Autodesk Inventor part; units mm, degrees
ref_plane "Work Plane1" through (0, -14.5, 0) normal (0, 1, 0) x (-1, 0, 0)
ref_plane "Work Plane2" through (0, 14.5, 0) normal (0, 1, 0) x (-1, 0, 0)
ref_plane "YZ Plane" through (0, 0, 0) normal (1, 0, 0) x (0, 1, 0)
sketch "Sketch2" plane through (0, 0, 0) normal (0, 1, 0) x (-1, 0, 0)
  circle A0 centre (-25, -83.5) radius 36 construction
  line L0 (-25, -83.5) -> (-61, -83.5) construction
  line L1 (-25, -83.5) -> (4.6941, -63.1466) construction
  circle A1 centre (-25, -83.5) radius 41.5
  circle A2 centre (-25, -83.5) radius 28
  arc A3 (-8.1325, -61.1508) -> (0, -50.3752) centre (-4.0663, -55.763) ccw
  arc A4 (-50, -50.3752) -> (-39.3017, -57.0193) centre (-45.9337, -55.763) ccw
  line L2 (-25, -83.5) -> (-4.0663, -55.763) construction
  circle A5 centre (-25, -83.5) radius 31.5
  line L3 (0, -50.3752) -> (0, 0)
  line L4 (-50, -50.3752) -> (-50, 0)
  line L5 (0, 0) -> (-50, 0)
  line L6 (-25, 0) -> (-25, -83.5) construction
  point P0 (15.9829, -76.969)
  point P1 (13.8342, -68.866)
  point P2 (-39.2078, -55.1936)
  point P3 (-41.8675, -61.1508)
  point P4 (-8.1325, -61.1508)
  dimension "d1" = 72
  dimension "d5" = 83
  dimension "d6" = 56
  dimension "d7" = 63
  dimension "d11" = 50
  dimension "d31" = 83.5
ref_plane "Work Plane1" through (0, -14.5, 0) normal (0, 1, 0) x (-1, 0, 0)
ref_plane "Work Plane2" through (0, 14.5, 0) normal (0, 1, 0) x (-1, 0, 0)
extrude "Extrusion1" add sketch "Sketch2" along normal blind 12 from surface at 14.5 contours A1 A4 A5 A3 | A3 A5 A4 A1
extrude "Extrusion2" add sketch "Sketch2" against normal blind 12 from surface at -14.5 contours A3 A5 A4 A1 | A3 A2 A4 A5 picked at (-44.9519, -51.1635) picked at (-38.3765, -56.444)
extrude "Extrusion3" add sketch "Sketch2" along normal mid plane 53 contours A1 L4 L5 L3
sketch "Sketch3" plane through (0, 0, 0) normal (1, 0, 0) x (0, 1, 0)
  line L0 (26.5, 0) -> (-26.5, 0)
  circle A0 centre (0, 0) radius 26.5
extrude "Extrusion4" add sketch "Sketch3" along normal up to surface (50 mm away)
properties part number "left_thigh"
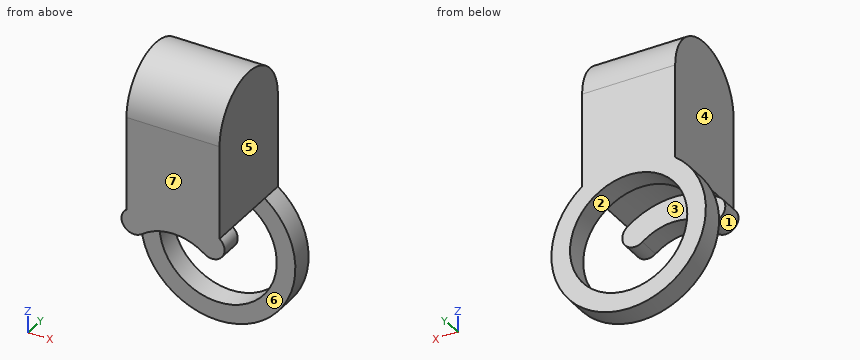
Design review of the part built by this model. Coordinates are the model's own, in mm. Face numbers are marked on the shaded views. A direction names the side the tool comes from. Coordinates: 2 decimals unless noted, no trailing zeros. Loops run counter-clockwise (first coordinate to the right, second up) from the corner with the lowest first, then second, coordinate; pieces in that order, holes last. Notation, with made-up numbers: M 64,20 L 115,20 A23 cw 115,30 Z; hole C -11,80.25 d5. An arc over 180 degrees is marked long. Answer as CSV lines item,"result".
Item 1: The part is to be moulded in two halves that separate along Y. For the marked faces 5, 6 and 7, say which applies: pulls with the +Y half, pulls with the -Y half, needs draft (parallel to the pull), parting line crosses it, or undercut.
Answer list:
face 5,"needs draft"
face 6,"undercut"
face 7,"pulls with the -Y half"
Item 2: Add section C-C on z = -46. State the section outline as (x, y) points.
Answer list:
outline,"M 0,-26.5 L 50,-26.5 L 50,26.5 L 0,26.5 Z; hole M 7.22,-14.5 L 42.78,-14.5 L 42.78,14.5 L 7.22,14.5 Z"
Item 3: Add section D-D on y = 18.5. State the section outline as (x, z) points, plus the area to 3 significant figures.
Answer list:
outline,"M 0,-50.38 A41.5 ccw long 50,-50.38 L 50,18.97 L 0,18.97 Z; hole C 25,-83.5 d63"
area,"5,480 mm²"
Item 4: Add section A-A on x = 25. State the section outline as (y, z) points.
Answer list:
outline,"M -26.5,-55.5 L -14.5,-55.5 L -14.5,-42 L 14.5,-42 L 14.5,-52 L 26.5,-52 L 26.5,0 A26.5 ccw -26.5,0 Z; M 14.5,-125 L 26.5,-125 L 26.5,-115 L 14.5,-115 Z"
Item 5: Add section B-B on z = -83.5. State the section outline as (x, y) points, plus the area to 3 significant figures.
Answer list:
outline,"M -16.5,14.5 L -6.5,14.5 L -6.5,26.5 L -16.5,26.5 Z; M 56.5,14.5 L 66.5,14.5 L 66.5,26.5 L 56.5,26.5 Z"
area,"240 mm²"
Item 6: Machinability: for the marked faces 1, 2, 3 and 4, which of the approach directions +Z, -Z, +X, -X, +Y, -Y give a long, thin tool a straight path to every point of the face, cutting with its end or side? Answer none if there is none.
Answer list:
face 1,"-Y"
face 2,"+Y"
face 3,"-Z"
face 4,"+Z, -X, +Y, -Y"
Item 7: For probe 1 along X at (y, z) = (18.25, -83.5); probe 2 along Y at (x, z) = (8.5, -48); probe 3 along X at (y, z) = (8.5, -21.5), list the stretches that pass through material, from the lowest coordinate up.
Answer list:
probe 1,"-16.5 to -6.5, 56.5 to 66.5"
probe 2,"-26.5 to -14.5, 14.5 to 26.5"
probe 3,"0 to 50"
Item 8: For P1, Ø2, axis at x = 14.5, y = 2.5, coming from the +Z side; P2, Ø16, axis at y = 5, z = 2.5, coming from the -X side; P3, Ø12, axis at y = 10.5, z = -31.5, coming from the +X side, all flat-tipped, find the tip position at first contact; note any pin that passes through.
Answer list:
P1,"z = 26.46"
P2,"x = 0"
P3,"x = 50"
